from build123d import *

# Parameters (mm, degrees)
SKETCH1_R           = 14
BOSS_EXTRUDE1_DEPTH = 4
SKETCH2_R           = 2.94
BOSS_EXTRUDE2_DEPTH = 9.7
SKETCH4_R           = 11
CUT_EXTRUDE1_DEPTH  = 1
FILLET1_R           = 0.5
FILLET2_R           = 1.5


with BuildPart() as part:
    # Sketch1 → Boss-Extrude1 (new body)
    with BuildSketch(Plane.XY):
        Circle(SKETCH1_R)
    extrude(amount=BOSS_EXTRUDE1_DEPTH)

    # Sketch2 → Boss-Extrude2 (add)
    with BuildSketch(Plane.XY.offset(4)):
        Circle(SKETCH2_R)
    extrude(amount=BOSS_EXTRUDE2_DEPTH)

    # Sketch4 → Cut-Extrude1 (cut)
    with BuildSketch(Plane(origin=(0, 0, 0), x_dir=(-1, 0, 0), z_dir=(0, 0, -1))):
        Circle(SKETCH4_R)
    extrude(amount=-CUT_EXTRUDE1_DEPTH, mode=Mode.SUBTRACT)

    # Fillet1
    fillet1_edges = [part.edges().sort_by_distance(p)[0] for p in [
        (11, 0, 1),
        (11, 0, 0),
    ]]
    fillet(fillet1_edges, radius=FILLET1_R - 0.0001)  # a hair under: the kernel refuses the full size

    # Fillet2
    fillet2_edges = [part.edges().sort_by_distance(p)[0] for p in [
        (-14, 0, 0),
    ]]
    fillet(fillet2_edges, radius=FILLET2_R)


solid = part.part
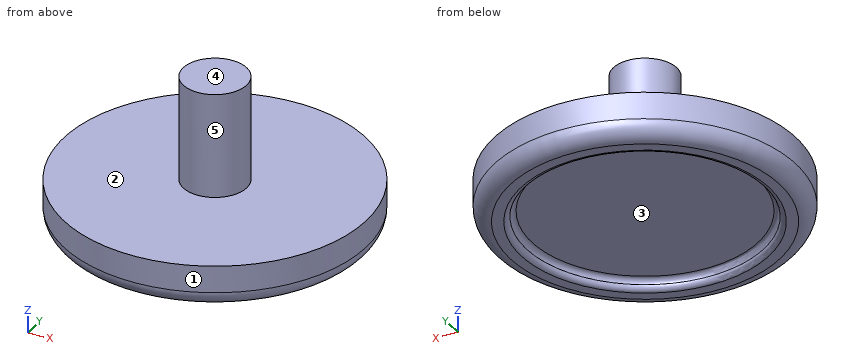
For this review, take the finished solid that the model builds, in its own axes (mm). Face numbers are marked on the shaded views. A direction names the side the tool comes from. Round coordinates to 2 decimals unless told otherwise and drop trailing zeros. Loops run counter-clockwise (first coordinate to the right, second up) from the corner with the lowest first, then second, coordinate; pieces in that order, holes last. Notation, with made-up numbers: (34.5, 54.5) - (46.5, 54.5) arc R19 cw to (46.5, 87.5) - close; hole circle Ø1 at (61, -19). An arc over 180 degrees is marked (long way). Put each result on its own line as item: value. Start each with the question number.
1. Mouldability with a two-part tool opening along Y and no side actions: class the marked faces 1, 2 and 3 as +Y half, -Y half, draft (parallel to the pull), parting line (faces both ways), or undercut.
2. For the marked faces 4 and 5, list the 3-axis set-ups (+Z, -Z, +X, -X, +Y, -Y) from which the entire face can be reached by the end or side of a thin tool; tool diameter is ignored.
3. Consider section D-D on z = 3. State the section outline as (x, y) points, plus the area to 3 significant figures.
4. Insertion check: P1, Ø2, axis at y = -3, z = 12, coming from the +X side; P2, Ø8, axis at x = -10, z = 2.5, coming from the -Y side; P3, Ø1.5, axis at x = 4.5, y = -2.5, coming from the +Z side. Each pin has a flat end and moves straight along its axis. Give the tip position at first contact, or say it passes through.
5. Consider section C-C on z = 5. State the section outline as (x, y) points, plus the area to 3 significant figures.
6. For probe 1 along Z at (x, y) = (-6.5, 6); probe 2 along Y at (x, z) = (0, 0.5); probe 3 along Y at (x, z) = (0, 0.55), list the stretches that pass through material, from the lowest coordinate up. Write a range as [from, to].
Result sheet:
1. face 1: parting line
1. face 2: draft
1. face 3: undercut
2. face 4: +Z, +X, -X, +Y, -Y
2. face 5: +Z
3. outline: circle Ø28 at (0, 0)
3. area: 616 mm^2
4. P1: x = 2.15
4. P2: y = -12.65
4. P3: z = 4
5. outline: circle Ø5.88 at (0, 0)
5. area: 27.2 mm^2
6. probe 1: [1, 4]
6. probe 2: [-13.62, -11], [11, 13.62]
6. probe 3: [-13.66, -11], [11, 13.66]
